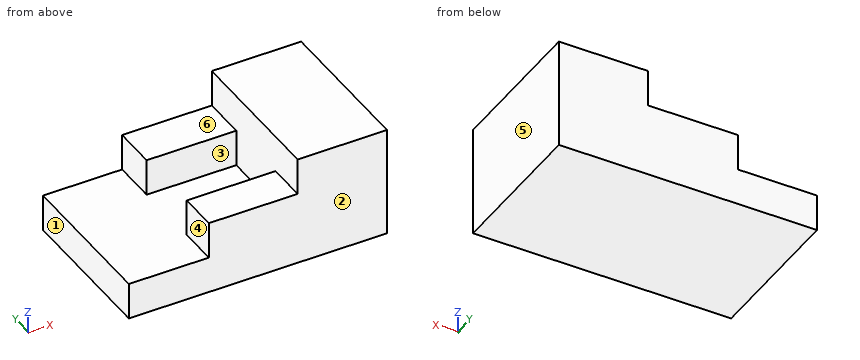
```python
from build123d import *

# Parameters (mm, degrees)
F0_W     = 88.9
F0_H     = 52.248245614
F1_DEPTH = 12.7
F2_W     = 30.8722835034
F2_H     = 14.9023200136
F2_W_2   = 30.5808074772
F2_H_2   = 13.4449426767
F3_DEPTH = 12.7
F4_DEPTH = 25.4


with BuildPart() as f1:
    # F0 (on Top) → F1 (new body)
    with BuildSketch(Plane.XY):
        Rectangle(F0_W, F0_H)
    extrude(amount=F1_DEPTH)

    # F2 (on face) → F3 (join)
    with BuildSketch(Plane.XY.offset(12.7)):
        with Locations((-1.7609084025, 18.6729628002)):
            Rectangle(F2_W, F2_H)
        with Locations((-1.6151703894, -19.4016514687)):
            Rectangle(F2_W_2, F2_H_2)
    extrude(amount=F3_DEPTH)

    # F2 (on face) → F4 (join)
    with BuildSketch(Plane.XY.offset(12.7)):
        Polygon((44.45, 26.124122807), (13.6752333492, 26.124122807), (13.6752333492, 11.2218027934), (13.6752333492, -12.6791801304), (13.6752333492, -26.124122807), (44.45, -26.124122807), (44.45, -12.6791801304), (44.45, 11.2218027934), align=None)
    extrude(amount=F4_DEPTH)


solid = f1.part
```
Work out the finished part from the listing and answer in its coordinate system (mm). Face numbers are marked on the shaded views. A direction names the side the tool comes from. Give positions to 0.01 mm unless a question says otherwise; leave off trailing zeros. Write each loop counter-clockwise with the first axis right and the second up, starting at its lowest first coordinate (ties: lowest second). Pieces come first, ordered by that corner, then holes. Notation, with made-up numbers: (38, 46) - (48, 46) arc R26 cw to (48, 76) - close; hole circle Ø2 at (-6, 25). An arc over 180 degrees is marked (long way). Use one line per item in the form item = value.
1. A cutting plane is placed at B-B (y = 22.5). Write down the section's boundary in (x, z).
Filled in:
outline = (-44.45, 0) - (44.45, 0) - (44.45, 38.1) - (13.68, 38.1) - (13.68, 25.4) - (-17.2, 25.4) - (-17.2, 12.7) - (-44.45, 12.7) - close
2. A cutting plane is placed at D-D (y = 8.5). Write down the section's boundary in (x, z), and give its area (3 significant figures).
Filled in:
outline = (-44.45, 0) - (44.45, 0) - (44.45, 38.1) - (13.68, 38.1) - (13.68, 12.7) - (-44.45, 12.7) - close
area = 1,910 mm^2
3. Determine the mould class of the marked faces 1, 2 and 3 for opening direction Y: released by +Y, released by -Y, zero draft, split by the parting line, or undercut.
Filled in:
face_1 = zero draft
face_2 = released by -Y
face_3 = undercut
4. Consider L1, parallel to Y at x = 10, z = 15; L2, parallel to Z at x = -15, y = 8.5; L3, parallel to X at y = -13, z = 31. Determine where each line is inside the solid, lowest interval first.
Filled in:
L1 = -26.12 to -12.68, 11.22 to 26.12
L2 = 0 to 12.7
L3 = 13.68 to 44.45
5. A cutting plane is placed at C-C (x = -27.5). Write down the section's boundary in (y, z), and give its area (3 significant figures).
Filled in:
outline = (-26.12, 0) - (26.12, 0) - (26.12, 12.7) - (-26.12, 12.7) - close
area = 664 mm^2
6. For the marked faces 4, 5 and 6, determine the directions among +Z, -Z, +X, -X, +Y, -Y from which every point of the face is accessible in a straight line to the end or side of a thin tool.
Filled in:
face_4 = +Z, -X, -Y
face_5 = +Z, -Z, +X, +Y, -Y
face_6 = +Z, -X, +Y, -Y
7. A cutting plane is placed at A-A (z = 24.5). Write down the section's boundary in (x, y), and give its area (3 significant figures).
Filled in:
outline = (-17.2, 11.22) - (13.68, 11.22) - (13.68, -12.68) - (-16.91, -12.68) - (-16.91, -26.12) - (44.45, -26.12) - (44.45, 26.12) - (-17.2, 26.12) - close
area = 2,480 mm^2
8. Each of these flat-tipped pins is pushed along its axis until it touches: pin 1 Ø5 at (y, z) = (18.5, 17.5) entering from -X; pin 2 Ø15 at (x, y) = (-7, -17.5) entering from +Z; pin 3 Ø12 at (x, y) = (-27.5, 16) entering from +Z. Where does it stop, or does it pass through?
Filled in:
pin_1 = -17.2
pin_2 = 25.4
pin_3 = 12.7
